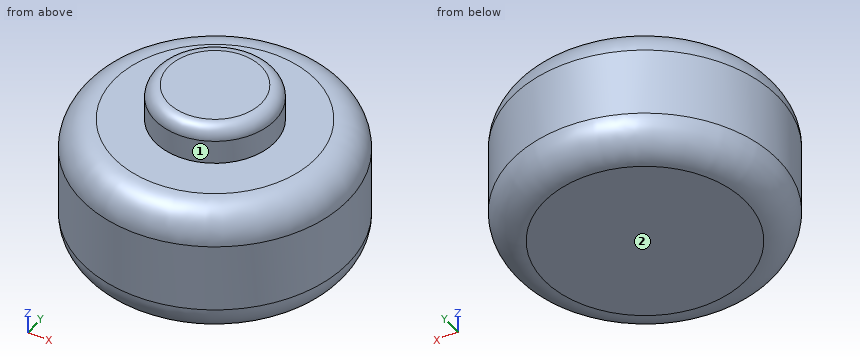
from build123d import *

# Parameters (mm, degrees)
F0_R     = 50
F1_DEPTH = 50
F2_R     = 12.071068
F3_R     = 22.5
F4_DEPTH = 14
F5_R     = 5


with BuildPart() as f1:
    # F0 (on Top) → F1 (new body)
    with BuildSketch(Plane.XY):
        Circle(F0_R)
    extrude(amount=F1_DEPTH)

    # F2
    f2_edges = [f1.edges().sort_by_distance(p)[0] for p in [
        (-50, 0, 50),
        (-50, 0, 0),
    ]]
    fillet(f2_edges, radius=F2_R)

    # F3 (on face) → F4 (join)
    with BuildSketch(Plane.XY.offset(50)):
        Circle(F3_R)
    extrude(amount=F4_DEPTH)

    # F5
    f5_edges = [f1.edges().sort_by_distance(p)[0] for p in [
        (-22.5, 0, 64),
    ]]
    fillet(f5_edges, radius=F5_R)


solid = f1.part
Can you work these out from the model? Positions are in its coordinate system, mm. Face numbers are marked on the shaded views. A direction names the side the tool comes from. Give positions to 0.01 mm unless a question says otherwise; leave off trailing zeros. Order: outer loops, then holes, each group sorted by start corner. A loop starts at its lowest first (then second) coordinate and runs counter-clockwise, first axis right, second up. Notation, with made-up numbers: M 42.25,-8 L 68.25,-8 A10 cw 68.25,10 Z; hole C -27,75.5 d10. An arc over 180 degrees is marked long. Use one line per item in the form item = value.
Item 1: If we section it at C-C, the plane z = 53.5: Write out the boundary of the cut face in (x, y), and give its area (3 significant figures).
Values follow:
outline = C 0,0 d45
area = 1,590 mm^2
Item 2: Will these pins go through, and if not, where does the flat tip stop? pin 1 Ø8 at (x, z) = (26, 52.5) entering from +Y; pin 2 Ø10 at (x, y) = (-33.5, 34) entering from +Z; pin 3 Ø5 at (x, z) = (-1.5, 20) entering from +Y.
Values follow:
pin_1 = 35.63
pin_2 = 49
pin_3 = 50
Item 3: If we section it at D-D, the plane z = 42: Write out the boundary of the cut face in (x, y), and give its area (3 significant figures).
Values follow:
outline = C 0,0 d98.59
area = 7,630 mm^2
Item 4: If I drill on line 1 along Z through (x, y) = (0, -27); line 2 along X through (y, z) = (-15, 13); line 3 along X through (y, z) = (-19.5, 15.5), over which ranges is the centre line in solid material (lowest first)? Write a range as [from, to].
Values follow:
line_1 = [0, 50]
line_2 = [-47.7, 47.7]
line_3 = [-46.04, 46.04]
Item 5: For the marked faces 1 and 2, which set-ups out of +Z, -Z, +X, -X, +Y, -Y let a thin tool reach every point of the face, with its end or its side?
Values follow:
face_1 = +Z
face_2 = -Z, +X, -X, +Y, -Y
Item 6: If we section it at A-A, the plane x = 0: Write out the boundary of the cut face in (y, z), and give its area (3 significant figures).
Values follow:
outline = M -50,12.07 A12.07 ccw -37.93,0 L 37.93,0 A12.07 ccw 50,12.07 L 50,37.93 A12.07 ccw 37.93,50 L 22.5,50 L 22.5,59 A5 ccw 17.5,64 L -17.5,64 A5 ccw -22.5,59 L -22.5,50 L -37.93,50 A12.07 ccw -50,37.93 Z
area = 5,490 mm^2
